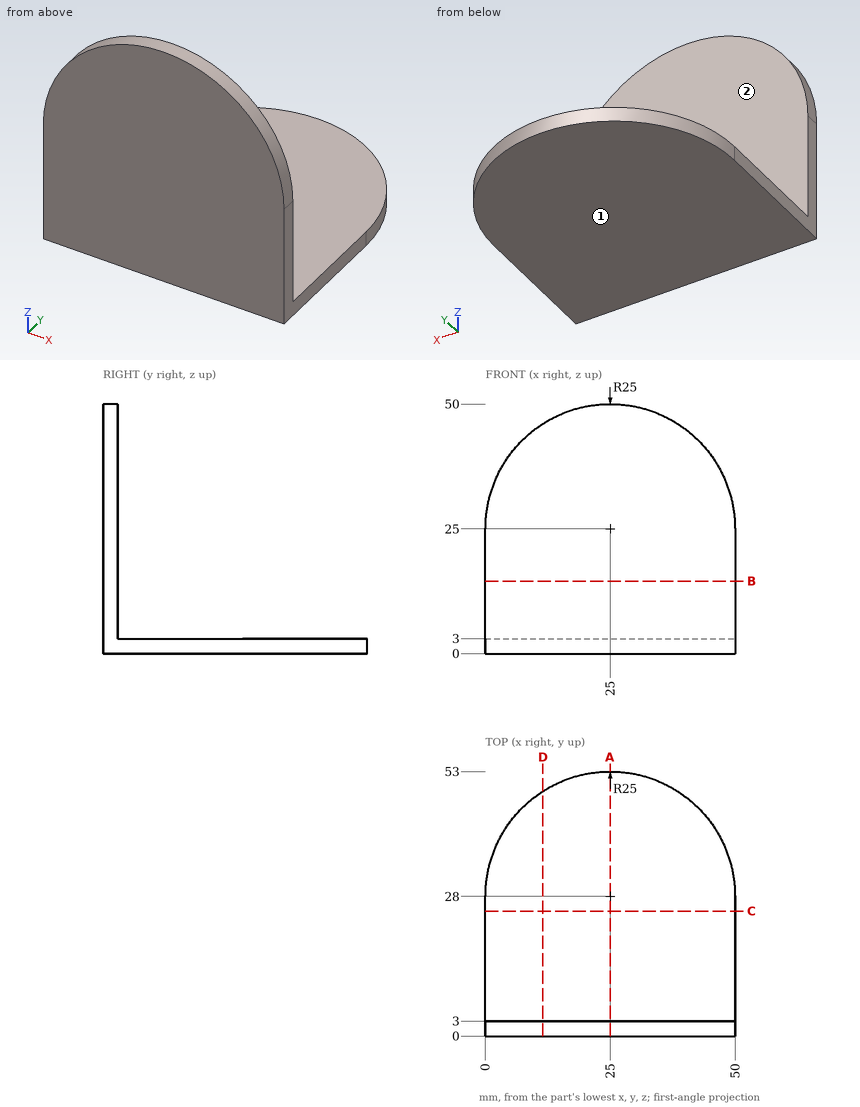
Check sheet for the drawn part. Datum: minimum x, y, z corner. Units: mm. A direction names the side the tool comes from. Coordinates: 2 decimals unless noted, no trailing zeros. Loops run counter-clockwise (first coordinate to the right, second up) from the corner with the lowest first, then second, coordinate; pieces in that order, holes last. Notation, with made-up numbers: (-20, -22.75) -> (24, -22.75) arc R11 ccw to (24, -17.75) -> close; hole circle Ø9 at (-6, -0.5). An arc over 180 degrees is marked (long way). Answer as a JSON object with one key per item and string values. Group by question number.
Item 1: Tool access check on the marked faces 1 and 2. Record the directions out of +Z, -Z, +X, -X, +Y, -Y that give a thin tool (end or side, any length) a straight path to the whole face; none if there is none.
Item 2: Sectioned sample at A-A on x = 25. Record the boundary of the cut face in (y, z), plus the area to 3 significant figures.
Item 3: Sectioned sample at D-D on x = 11.5. Record the boundary of the cut face in (y, z), plus the area to 3 significant figures.
Item 4: Scan line: probe 1 along Y at (x, z) = (18.5, 26.5). Record every from-to range of solid material in increasing order.
Item 5: Depth check by flat-ended pin: pin 1 (1 mm diameter, centred on x = 18.5, y = 26, fed in from +Z); pin 2 (5 mm diameter, centred on x = 24.5, z = 26, fed in from +Y). Enter the tip coordinate at first touch or a pass-through.
Item 6: Sectioned sample at B-B on z = 14.5. Record the boundary of the cut face in (x, y), plus the area to 3 significant figures.
Evaluation:
{
 "1": {"face 1": "-Z, +X, -X, +Y, -Y", "face 2": "+Z, +X, -X, +Y"},
 "2": {"outline": "(0, 0) -> (53, 0) -> (53, 3) -> (3, 3) -> (3, 50) -> (0, 50) -> close", "area": "300 mm²"},
 "3": {"outline": "(0, 0) -> (49.04, 0) -> (49.04, 3) -> (3, 3) -> (3, 46.04) -> (0, 46.04) -> close", "area": "276 mm²"},
 "4": {"probe 1": "y = 0 to 3"},
 "5": {"pin 1": "stops at z = 3", "pin 2": "stops at y = 3"},
 "6": {"outline": "(0, 0) -> (50, 0) -> (50, 3) -> (0, 3) -> close", "area": "150 mm²"}
}
